```python
from build123d import *

# Parameters (mm, degrees)
EXTRUDE_1_DEPTH     = 10
SKETCH_2_W          = 20
SKETCH_2_H          = 14
EXTRUDE_2_DEPTH     = 10
CUT_EXTRUDE_1_REACH = 29.536
SKETCH_3_R          = 4
SKETCH_3_R_2        = 2.75
CUT_EXTRUDE_2_REACH = 29.536
SKETCH_4_W          = 1.5
SKETCH_4_H          = 14


with BuildPart() as part:
    # 草图1 → 凸台-拉伸1 (new body)
    with BuildSketch(Plane.XY):
        with BuildLine():
            Line((-17.646494004, -5.247766906), (-2.5, -10))
            Line((-2.5, -10), (2.5, -10))
            Line((2.5, -10), (17.646494004, -5.247766906))
            ThreePointArc((17.646494004, -5.247766906), (21.5, 0), (17.646494004, 5.247766906))
            Line((17.646494004, 5.247766906), (2.5, 10))
            Line((2.5, 10), (-2.5, 10))
            Line((-2.5, 10), (-17.646494004, 5.247766906))
            ThreePointArc((-17.646494004, 5.247766906), (-21.5, 0), (-17.646494004, -5.247766906))
        make_face()
    extrude(amount=EXTRUDE_1_DEPTH)

    # 草图2 → 凸台-拉伸2 (add)
    with BuildSketch(Plane.XY.offset(10)):
        with Locations((0, -7)):
            Rectangle(SKETCH_2_W, SKETCH_2_H)
    extrude(amount=-EXTRUDE_2_DEPTH)

    # 草图3 → 切除-拉伸1 (cut, up to next)
    with BuildSketch(Plane.XY.offset(10), mode=Mode.PRIVATE) as cut_extrude_1_sk1:
        Circle(SKETCH_3_R)
    cut_extrude_1_tool1 = extrude(cut_extrude_1_sk1.sketch, amount=-CUT_EXTRUDE_1_REACH, mode=Mode.PRIVATE) & part.part
    # 草图3 → 切除-拉伸1 (cut, up to next)
    with BuildSketch(Plane.XY.offset(10), mode=Mode.PRIVATE) as cut_extrude_1_sk2:
        with Locations((-16, 0)):
            Circle(SKETCH_3_R_2)
    cut_extrude_1_tool2 = extrude(cut_extrude_1_sk2.sketch, amount=-CUT_EXTRUDE_1_REACH, mode=Mode.PRIVATE) & part.part
    # 草图3 → 切除-拉伸1 (cut, up to next)
    with BuildSketch(Plane.XY.offset(10), mode=Mode.PRIVATE) as cut_extrude_1_sk3:
        with Locations((16, 0)):
            Circle(SKETCH_3_R_2)
    cut_extrude_1_tool3 = extrude(cut_extrude_1_sk3.sketch, amount=-CUT_EXTRUDE_1_REACH, mode=Mode.PRIVATE) & part.part
    add(cut_extrude_1_tool1.solids().sort_by_distance((0, 0, 10))[0], mode=Mode.SUBTRACT)
    add(cut_extrude_1_tool2.solids().sort_by_distance((-16, 0, 10))[0], mode=Mode.SUBTRACT)
    add(cut_extrude_1_tool3.solids().sort_by_distance((16, 0, 10))[0], mode=Mode.SUBTRACT)

    # 草图4 → 切除-拉伸2 (cut, up to next)
    with BuildSketch(Plane.XY.offset(10), mode=Mode.PRIVATE) as cut_extrude_2_sk1:
        with Locations((0, -7)):
            Rectangle(SKETCH_4_W, SKETCH_4_H)
    cut_extrude_2_tool1 = extrude(cut_extrude_2_sk1.sketch, amount=-CUT_EXTRUDE_2_REACH, mode=Mode.PRIVATE) & part.part
    add(cut_extrude_2_tool1.solids().sort_by_distance((0, -7, 10))[0], mode=Mode.SUBTRACT)


solid = part.part
```
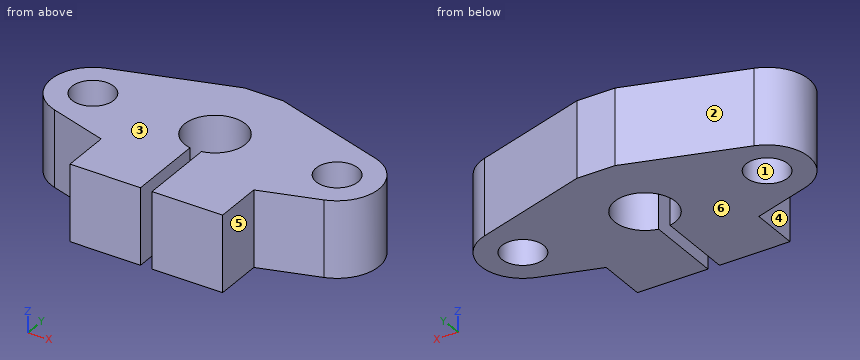
Build history of the part. All positions in model axes, mm. Face numbers are marked on the shaded views. A direction names the side the tool comes from. Round coordinates to 2 decimals unless told otherwise and drop trailing zeros. Write each loop counter-clockwise with the first axis right and the second up, starting at its lowest first coordinate (ties: lowest second). Pieces come first, ordered by that corner, then holes.
1) Mould opens along X. For the marked faces 1, 2 and 3 say: +X half, -X half, draft (parallel to the pull), parting line (faces both ways), or undercut.
2) Drill centre lines: probe 1 along X at (y, z) = (-1.75, 7.5); probe 2 along X at (y, z) = (0.75, 1.5); probe 3 along X at (y, z) = (-10.75, 3). Where is each one in solid material? Low to high.
3) Band-saw the part on C-C, the plane y = -8.75. List the corners of the cut face in (x, z).
4) 3-axis set-ups, long thin cutter, end or side, ignore diameter. For the marked faces 4, 5 and 6: which of +Z, -Z, +X, -X, +Y, -Y reach the whole face in a straight line?
5) Band-saw the part on B-B, the plane x = 17. List the corners of the cut face in (y, z).
6) Band-saw the part on D-D, the plane z = 8. List the corners of the cut face in (x, y), and give its area (3 significant figures).
7) Band-saw the part on A-A, the plane y = 0. List the corners of the cut face in (x, z), and give its area (3 significant figures).
8) Pin check, flat tips, straight feed: pin 1 (1.5 mm diameter, centred on x = 10.5, z = 7.5, fed in from +Y); pin 2 (3 mm diameter, centred on y = -12, z = 3, fed in from -X); pin 3 (6 mm diameter, centred on y = -11.5, z = 1.5, fed in from +X). Stop position of each tip, or through.
Ans:
1. face 1: undercut
1. face 2: -X half
1. face 3: draft
2. probe 1: x = -21.21 to -18.12, -13.88 to -3.6, 3.6 to 13.88, 18.12 to 21.21
2. probe 2: x = -21.45 to -18.65, -13.35 to -3.93, 3.93 to 13.35, 18.65 to 21.45
2. probe 3: x = -10 to -0.75, 0.75 to 10
3. outline: (-10, 0) - (-0.75, 0) - (-0.75, 10) - (-10, 10) - close; (0.75, 0) - (10, 0) - (10, 10) - (0.75, 10) - close
4. face 4: +Z, -Z, -X, -Y
4. face 5: +Z, -Z, +X, -Y
4. face 6: -Z, +X, -X, +Y, -Y
5. outline: (-5.45, 0) - (-2.56, 0) - (-2.56, 10) - (-5.45, 10) - close; (2.56, 0) - (5.45, 0) - (5.45, 10) - (2.56, 10) - close
6. outline: (-17.65, -5.25) - (-10, -7.65) - (-10, -14) - (-0.75, -14) - (-0.75, -3.93) arc R4 cw (long way) to (0.75, -3.93) - (0.75, -14) - (10, -14) - (10, -7.65) - (17.65, -5.25) arc R5.5 ccw to (17.65, 5.25) - (2.5, 10) - (-2.5, 10) - (-17.65, 5.25) arc R5.5 ccw to start; hole circle Ø5.5 at (-16, 0); hole circle Ø5.5 at (16, 0)
6. area: 606 mm2
7. outline: (-21.5, 0) - (-18.75, 0) - (-18.75, 10) - (-21.5, 10) - close; (-13.25, 0) - (-4, 0) - (-4, 10) - (-13.25, 10) - close; (4, 0) - (13.25, 0) - (13.25, 10) - (4, 10) - close; (18.75, 0) - (21.5, 0) - (21.5, 10) - (18.75, 10) - close
7. area: 240 mm2
8. pin 1: stops at y = 7.73
8. pin 2: stops at x = -10
8. pin 3: stops at x = 10
